Autodesk Inventor part; units mm, degrees
ref_plane "YZ Plane" through (0, 0, 0) normal (1, 0, 0) x (0, 1, 0)
ref_plane "XZ Plane" through (0, 0, 0) normal (0, 1, 0) x (-1, 0, 0)
ref_plane "XY Plane" through (0, 0, 0) normal (0, 0, 1) x (1, 0, 0)
sketch "Sketch1" plane through (0, 0, 0) normal (0, 0, 1) x (1, 0, 0)
  line L0 (-23.6052, 15.8968) -> (1.3948, 15.8968)
  line L1 (1.3948, 15.8968) -> (1.3948, 0.4466)
  line L2 (1.3948, 0.4466) -> (-23.6052, 0.4466)
  line L3 (-23.6052, 0.4466) -> (-23.6052, 15.4466)
  line L4 (-23.6052, 15.8968) -> (-26.1052, 15.8968)
  line L5 (-25.6052, 15.7466) -> (-25.6052, 15.4466)
  line L6 (-25.6052, 15.4466) -> (-23.6052, 15.4466)
  line L7 (-26.1052, 15.8968) -> (-26.6052, 15.8968)
  line L8 (-26.6052, 15.8968) -> (-26.6052, 15.7466)
  line L9 (-26.6052, 15.7466) -> (-25.6052, 15.7466)
  point P0 (0, 0)
  dimension "d0" = 15
  dimension "d1" = 25
  dimension "d2" = 2
  dimension "d3" = 1
  dimension "d4" = 2.5
  dimension "d5" = 0.5
  dimension "d6" = 0.1502
  dimension "d7" = 0.3
extrude "Extrusion1" add sketch "Sketch1" along normal blind 35
sketch "Sketch4" plane through (0, 0, 35) normal (0, 0, 1) x (1, 0, 0)
  line L0 (-26.6052, 15.8968) -> (-26.6052, 15.7466)
  line L1 (-26.6052, 15.7466) -> (-25.6052, 15.7466)
  line L2 (-25.6052, 15.7466) -> (-25.6052, 15.4466)
  line L3 (-25.6052, 15.4466) -> (-23.6052, 15.4466)
  line L4 (-23.6052, 15.4466) -> (-23.6052, 0.4466)
  line L5 (-23.6052, 0.4466) -> (1.3948, 0.4466)
  line L6 (1.3948, 0.4466) -> (1.3948, 15.8968)
  line L7 (1.3948, 15.8968) -> (-26.6052, 15.8968)
  line L8 (-16.9052, 11.8968) -> (-16.1052, 11.8968)
  line L9 (-16.1052, 11.8968) -> (-16.1052, 11.0968)
  line L10 (-16.1052, 11.0968) -> (-16.9052, 11.0968)
  line L11 (-16.9052, 11.0968) -> (-16.9052, 11.8968)
  line L12 (-23.6052, 0.4466) -> (1.3948, 0.4466)
  line L13 (-11.1052, 0.4466) -> (-11.1052, 15.8968)
  line L14 (1.3948, 15.8968) -> (-26.6052, 15.8968)
  line L15 (-5.3052, 11.8968) -> (-6.1052, 11.8968)
  line L16 (-6.1052, 11.8968) -> (-6.1052, 11.0968)
  line L17 (-6.1052, 11.0968) -> (-5.3052, 11.0968)
  line L18 (-5.3052, 11.0968) -> (-5.3052, 11.8968)
  point P0 (0, 0)
  dimension "d26" = 10
  dimension "d27" = 0.8
  dimension "d28" = 0.8
  dimension "d29" = 4
extrude "Extrusion2" cut sketch "Sketch4" against normal blind 1 contours L8 L9 L10 L11 | L18 L17 L16 L15
sketch "Sketch5" plane through (-23.6052, 0.4466, 0) normal (-1, 0, 0) x (0, 0, 1)
  line L0 (0, 15) -> (0, 0)
  line L1 (0, 0) -> (35, 0)
  line L2 (35, 15) -> (35, 0)
  line L3 (0, 15) -> (35, 15)
  line L4 (12, 5) -> (15, 5)
  line L5 (15, 5) -> (15, 4)
  line L6 (15, 4) -> (12, 4)
  line L7 (12, 4) -> (12, 5)
  point P0 (0, -0.4466)
  dimension "d32" = 1
  dimension "d33" = 3
  dimension "d34" = 10
  dimension "d35" = 20
extrude "Extrusion3" cut sketch "Sketch5" against normal blind 1 contours L4 L5 L6 L7
equation "\"d28\" = d27"
properties part number "McCrea_zadne_oko_walle" material "Silver"
The listing builds one solid part. Answer for the finished solid, in the listing's coordinates (mm). A direction names the side the tool comes from. Give positions to 0.01 mm unless a question says otherwise; leave off trailing zeros. Loops run counter-clockwise (first coordinate to the right, second up) from the corner with the lowest first, then second, coordinate; pieces in that order, holes last. Notation, with made-up numbers: M -39,75 L -24,75 A34 cw -24,107 Z; hole C 7,59 d9. An arc over 180 degrees is marked long. One line per item, written item: value.
1. Each of these flat-tipped pins is pushed along its axis until it touches: P1, Ø0.6, axis at x = -6, y = 11.5, coming from the +Z side; P2, Ø4.5, axis at y = 6.5, z = 24, coming from the -X side; P3, Ø0.5, axis at y = 5, z = 13, coming from the -X side. Where does it stop, or does it pass through?
Found:
P1: z = 35
P2: x = -23.61
P3: x = -22.61
2. Section A-A on y = 5 is taken. Determine the outline of the cut face in (x, z), plus the area to 3 significant figures.
Found:
outline: M -23.61,0 L 1.39,0 L 1.39,35 L -23.61,35 L -23.61,15 L -22.61,15 L -22.61,12 L -23.61,12 Z
area: 872 mm^2
3. For faces 1 (the face through (-23, 5, 15)), 2 (the face through (-16.105, 11.5, 34.5)), 3 (the face through (-13, 8, 35)), 4 (the face through (-25, 15.447, 17)), determine the directions among +Z, -Z, +X, -X, +Y, -Y from which every point of the face is accessible in a straight line to the end or side of a thin tool.
Found:
face 1: -X
face 2: +Z
face 3: +Z, +X, -X, +Y, -Y
face 4: +Z, -Z, -X, -Y
4. For a pull along Y with two mould halves and no side action, classify faces 5 (the face through (-11, 0.447, 17)), 6 (the face through (-13, 15.897, 17)), 7 (the face through (-13, 8, 0)), 8 (the face through (-16.5, 11.5, 34)) as pulls with the +Y half, pulls with the -Y half, needs draft (parallel to the pull), parting line crosses it, or undercut.
Found:
face 5: pulls with the -Y half
face 6: pulls with the +Y half
face 7: needs draft
face 8: undercut
5. Section D-D on z = 13.5 is taken. Determine the outline of the cut face in (x, y), plus the area to 3 significant figures.
Found:
outline: M -26.61,15.75 L -25.61,15.75 L -25.61,15.45 L -23.61,15.45 L -23.61,5.45 L -22.61,5.45 L -22.61,4.45 L -23.61,4.45 L -23.61,0.45 L 1.39,0.45 L 1.39,15.9 L -26.61,15.9 Z
area: 386 mm^2
6. Section C-C on x = -24.5 is taken. Determine the outline of the cut face in (y, z).
Found:
outline: M 15.45,0 L 15.9,0 L 15.9,35 L 15.45,35 Z
7. Section B-B on z = 31.5 is taken. Determine the outline of the cut face in (x, y).
Found:
outline: M -26.61,15.75 L -25.61,15.75 L -25.61,15.45 L -23.61,15.45 L -23.61,0.45 L 1.39,0.45 L 1.39,15.9 L -26.61,15.9 Z
8. Find the intervals of material crossed by probe 1 along X at (y, z) = (13.25, 11), in increasing order.
Found:
probe 1: -23.61 to 1.39
